from build123d import *

# Parameters (mm, degrees)
SKETCH1_W               = 50
SKETCH1_H               = 50
BOSS_EXTRUDE1_DEPTH     = 12
FILLET1_R               = 5
SKETCH3_R               = 18.25
CUT_EXTRUDE1_DEPTH      = 5.5
SKETCH4_R               = 11.25
CUT_EXTRUDE2_DEPTH      = 10
SKETCH5_W               = 62.97921445
SKETCH5_H               = 70.453436458
CUT_EXTRUDE3_DEPTH      = 3
SKETCH6_R               = 2.5
CUT_EXTRUDE4_DEPTH      = 2
SKETCH7_R               = 1.55
CUT_EXTRUDE5_DEPTH      = 3
SKETCH8_R               = 1.55
CUT_EXTRUDE6_DEPTH      = 12
SKETCH9_R               = 3.75
CUT_EXTRUDE7_DEPTH      = 5
MIRROR2_COPY_1_SKETCH_R = 1.55
MIRROR2_COPY_1_DEPTH    = 12
MIRROR2_COPY_2_SKETCH_R = 3.75
MIRROR2_COPY_2_DEPTH    = 5


with BuildPart() as part:
    # Sketch1 → Boss-Extrude1 (new body)
    with BuildSketch(Plane(origin=(0, 0, 0), x_dir=(1, 0, 0), z_dir=(0, 1, 0))):
        Rectangle(SKETCH1_W, SKETCH1_H)
    extrude(amount=BOSS_EXTRUDE1_DEPTH)

    # Fillet1
    fillet1_edges = [part.edges().sort_by_distance(p)[0] for p in [
        (25, 6, 25),
        (-25, 6, 25),
        (-25, 6, -25),
        (25, 6, -25),
    ]]
    fillet(fillet1_edges, radius=FILLET1_R)

    # Sketch3 → Cut-Extrude1 (cut)
    with BuildSketch(Plane.XZ):
        Circle(SKETCH3_R)
    extrude(amount=-CUT_EXTRUDE1_DEPTH, mode=Mode.SUBTRACT)

    # Sketch4 → Cut-Extrude2 (cut)
    with BuildSketch(Plane.XZ.offset(-5.5)):
        Circle(SKETCH4_R)
    extrude(amount=-CUT_EXTRUDE2_DEPTH, mode=Mode.SUBTRACT)

    # Sketch5 → Cut-Extrude3 (cut)
    with BuildSketch(Plane(origin=(0, 12, 0), x_dir=(1, 0, 0), z_dir=(0, 1, 0))):
        Rectangle(SKETCH5_W, SKETCH5_H)
    extrude(amount=-CUT_EXTRUDE3_DEPTH, mode=Mode.SUBTRACT)

    # Sketch6 → Cut-Extrude4 (cut)
    with BuildSketch(Plane(origin=(0, 9, 0), x_dir=(1, 0, 0), z_dir=(0, 1, 0))):
        with Locations((-9.899494937, 9.899494937)):
            Circle(SKETCH6_R)
        with Locations((9.899494937, 9.899494937)):
            Circle(SKETCH6_R)
        with Locations((-9.899494937, -9.899494937)):
            Circle(SKETCH6_R)
        with Locations((9.899494937, -9.899494937)):
            Circle(SKETCH6_R)
    extrude(amount=-CUT_EXTRUDE4_DEPTH, mode=Mode.SUBTRACT)

    # Sketch7 → Cut-Extrude5 (cut)
    with BuildSketch(Plane(origin=(0, 7, 0), x_dir=(1, 0, 0), z_dir=(0, 1, 0))):
        with Locations((-9.899494937, 9.899494937)):
            Circle(SKETCH7_R)
        with Locations((9.899494937, 9.899494937)):
            Circle(SKETCH7_R)
        with Locations((-9.899494937, -9.899494937)):
            Circle(SKETCH7_R)
        with Locations((9.899494937, -9.899494937)):
            Circle(SKETCH7_R)
    extrude(amount=-CUT_EXTRUDE5_DEPTH, mode=Mode.SUBTRACT)

    # Sketch8 → Cut-Extrude6 (cut)
    with BuildSketch(Plane(origin=(0, 9, 0), x_dir=(1, 0, 0), z_dir=(0, 1, 0))):
        with Locations((-22, 21.6)):
            Circle(SKETCH8_R)
    cut_extrude6 = extrude(amount=-CUT_EXTRUDE6_DEPTH, mode=Mode.SUBTRACT)

    # Sketch9 → Cut-Extrude7 (cut)
    with BuildSketch(Plane(origin=(0, 9, 0), x_dir=(1, 0, 0), z_dir=(0, 1, 0))):
        with Locations((-22, 21.6)):
            Circle(SKETCH9_R)
    cut_extrude7 = extrude(amount=-CUT_EXTRUDE7_DEPTH, mode=Mode.SUBTRACT)

    # Mirror1: Cut-Extrude6, Cut-Extrude7 across plane
    add(cut_extrude6.mirror(Plane(origin=(0, 0, 0), x_dir=(0, 0, 1), z_dir=(1, 0, 0))), mode=Mode.SUBTRACT)
    add(cut_extrude7.mirror(Plane(origin=(0, 0, 0), x_dir=(0, 0, 1), z_dir=(1, 0, 0))), mode=Mode.SUBTRACT)

    # Mirror2: Cut-Extrude6, Cut-Extrude7 across plane
    add(cut_extrude6.mirror(Plane.XY), mode=Mode.SUBTRACT)
    add(cut_extrude7.mirror(Plane.XY), mode=Mode.SUBTRACT)

    # Mirror2 copy 1 sketch → Mirror2 copy 1 (cut)
    with BuildSketch(Plane(origin=(0, 9, 0), x_dir=(-1, 0, 0), z_dir=(0, 1, 0))):
        with Locations((-22, 21.6)):
            Circle(MIRROR2_COPY_1_SKETCH_R)
    extrude(amount=-MIRROR2_COPY_1_DEPTH, mode=Mode.SUBTRACT)

    # Mirror2 copy 2 sketch → Mirror2 copy 2 (cut)
    with BuildSketch(Plane(origin=(0, 9, 0), x_dir=(-1, 0, 0), z_dir=(0, 1, 0))):
        with Locations((-22, 21.6)):
            Circle(MIRROR2_COPY_2_SKETCH_R)
    extrude(amount=-MIRROR2_COPY_2_DEPTH, mode=Mode.SUBTRACT)


solid = part.part
Here's how the part is built. I have some questions about the finished solid (model axes, mm). A direction names the side the tool comes from. Coordinates: 2 decimals unless noted, no trailing zeros. Write each loop counter-clockwise with the first axis right and the second up, starting at its lowest first coordinate (ties: lowest second). Pieces come first, ordered by that corner, then holes.
1) If we section it at D-D (x = -10): List the corners of the cut face in (y, z) for me.
Filled in:
outline: (0, -25) - (9, -25) - (9, -12.4) - (7, -12.4) - (7, -11.45) - (5.5, -11.45) - (5.5, -15.27) - (0, -15.27) - close; (0, 15.27) - (5.5, 15.27) - (5.5, 11.45) - (7, 11.45) - (7, 12.4) - (9, 12.4) - (9, 25) - (0, 25) - close; (5.5, -8.35) - (7, -8.35) - (7, -7.4) - (9, -7.4) - (9, -5.15) - (5.5, -5.15) - close; (5.5, 5.15) - (9, 5.15) - (9, 7.4) - (7, 7.4) - (7, 8.35) - (5.5, 8.35) - close
2) If we section it at B-B (z = 0): List the corners of the cut face in (x, y) for me, plus the area to 4 significant figures.
Filled in:
outline: (-25, 0) - (-18.25, 0) - (-18.25, 5.5) - (-11.25, 5.5) - (-11.25, 9) - (-25, 9) - close; (11.25, 5.5) - (18.25, 5.5) - (18.25, 0) - (25, 0) - (25, 9) - (11.25, 9) - close
area: 170.5 mm2
3) Which directions (+Z, -Z, +X, -X, +Y, -Y) give clear straight access to the entire face, cutting with the end or side of a thin tool? Please do faces 1 (the face through (8.669, 6.26, 10.843)), 2 (the face through (-19.16, 6.54, -19.15)), 3 (the face through (7.9, 5.5, 8.4)).
Filled in:
face 1: +Y, -Y
face 2: +Y
face 3: -Y
4) If we section it at A-A (x = 0): List the corners of the cut face in (y, z) for me.
Filled in:
outline: (0, -25) - (9, -25) - (9, -11.25) - (5.5, -11.25) - (5.5, -18.25) - (0, -18.25) - close; (0, 18.25) - (5.5, 18.25) - (5.5, 11.25) - (9, 11.25) - (9, 25) - (0, 25) - close
5) If I drill on line 1 (X direction, y = 7.5, z = -9); line 2 (Z direction, x = 0.5, y = 6.75); line 3 (Y direction, x = -10.5, z = 12.5), over which ranges is the centre line in solid material (lowest first)?
Filled in:
line 1: x = -25 to -12.23, -7.57 to -6.75, 6.75 to 7.57, 12.23 to 25
line 2: z = -25 to -11.24, 11.24 to 25
line 3: y = 5.5 to 9
6) I'm going to push flat-ended pins straight in: pin 1 (1.9 mm diameter, centred on x = 22, z = -21.6, fed in from -Y); pin 2 (4 mm diameter, centred on x = 9.9, z = 9.9, fed in from -Y); pin 3 (6 mm diameter, centred on x = -22, z = -21.6, fed in from +Y); pin 4 (4 mm diameter, centred on x = -9.9, z = -9.9, fed in from +Y). Where does each tip first touch, or does it pass through?
Filled in:
pin 1: passes through
pin 2: stops at y = 5.5
pin 3: stops at y = 4
pin 4: stops at y = 7
7) If we section it at C-C (y = 0.75): List the corners of the cut face in (x, z) for me.
Filled in:
outline: (-25, -20) arc R5 ccw to (-20, -25) - (20, -25) arc R5 ccw to (25, -20) - (25, 20) arc R5 ccw to (20, 25) - (-20, 25) arc R5 ccw to (-25, 20) - close; hole circle Ø3.1 at (-22, -21.6); hole circle Ø3.1 at (-22, 21.6); hole circle Ø36.5 at (0, 0); hole circle Ø3.1 at (22, -21.6); hole circle Ø3.1 at (22, 21.6)
